Here's how the part is built. I have some questions about the finished solid (model axes, mm). A direction names the side the tool comes from. Round coordinates to 2 decimals unless told otherwise and drop trailing zeros. Loops run counter-clockwise (first coordinate to the right, second up) from the corner with the lowest first, then second, coordinate; pieces in that order, holes last. Notation, with made-up numbers: M 33.5,7.5 L 88.5,7.5 A26 cw 88.5,27.5 Z; hole C -3,-8 d11. An arc over 180 degrees is marked long. Write each question's results on one line, items separated by ' | '. Start each with the question number.
```python
from build123d import *

# Parameters (mm, degrees)
EXTRUDE_1_DEPTH     = 40
CUT_EXTRUDE_1_DEPTH = 47.165463282
SKETCH_4_R          = 2
CUT_EXTRUDE_2_DEPTH = 47.165463282
SKETCH_5_W          = 15
SKETCH_5_H          = 15
EXTRUDE_2_DEPTH     = 17.5


with BuildPart() as part:
    # 草图1 → 凸台-拉伸1 (new body)
    with BuildSketch(Plane.XY):
        Polygon((0, 0), (15, 0), (15, -4), (-4, -4), (-4, 17.5), (0, 17.5), align=None)
    extrude(amount=EXTRUDE_1_DEPTH)

    # 草图2 → 切除-拉伸1 (cut, through all)
    with BuildSketch(Plane(origin=(0, 0, 0), x_dir=(1, 0, 0), z_dir=(0, 1, 0))):
        with BuildLine():
            Line((9.5, -36.5), (5.5, -36.5))
            ThreePointArc((5.5, -36.5), (4, -35), (5.5, -33.5))
            Line((5.5, -33.5), (9.5, -33.5))
            ThreePointArc((9.5, -33.5), (11, -35), (9.5, -36.5))
        make_face()
        with BuildLine():
            Line((9.5, -3.5), (5.5, -3.5))
            ThreePointArc((5.5, -3.5), (4, -5), (5.5, -6.5))
            Line((5.5, -6.5), (9.5, -6.5))
            ThreePointArc((9.5, -6.5), (11, -5), (9.5, -3.5))
        make_face()
    extrude(amount=-CUT_EXTRUDE_1_DEPTH, mode=Mode.SUBTRACT)

    # 草图4 → 切除-拉伸2 (cut, through all)
    with BuildSketch(Plane(origin=(0, 0, 0), x_dir=(0, 0, -1), z_dir=(1, 0, 0))):
        with Locations((-35, 8.75)):
            Circle(SKETCH_4_R)
        with Locations(Location((-5, 8.75, 0), (0, 0, 180))):
            Circle(SKETCH_4_R)
    extrude(amount=-CUT_EXTRUDE_2_DEPTH, mode=Mode.SUBTRACT)

    # 草图5 → 凸台-拉伸2 (add)
    with BuildSketch(Plane(origin=(0, 0, 0), x_dir=(1, 0, 0), z_dir=(0, 1, 0))):
        with Locations((7.5, -20)):
            Rectangle(SKETCH_5_W, SKETCH_5_H)
    extrude(amount=EXTRUDE_2_DEPTH)


solid = part.part
```
1. I want a section at D-D on x = 7.5. List the corners of the cut face in (y, z) for me.
2. I want a section at A-A on z = 5. List the corners of the cut face in (x, y) for me, plus the area to 3 significant figures.
3. I need wall thicknesses on line 1 along Y through (x, z) = (-1.2, 35); line 2 along X through (y, z) = (3.5, 2); line 3 along Z through (x, y) = (13.5, 4.5). Which ranges of each line are inside material? Lowest first, please.
4. If we mould it in two halves opening along X, with no side actions, what happens to faces 5 (the face through (-4, 7, 20)), 6 (the face through (11, -2, 35)), 7 (the face through (7, 0, 32))? For each: released by +X, released by -X, zero draft, split by the parting line, or undercut.
5. For pin 1 (3 mm diameter, centred on x = 8.5, y = -2.5, fed in from -Z); pin 2 (4 mm diameter, centred on x = 10, z = 5, fed in from +Y); pin 3 (10 mm diameter, centred on y = 10, z = 6, fed in from +X); pin 4 (4.5 mm diameter, centred on x = 9, y = 10, fed in from +Z), each with a flat end and sliding along its axis, tell me the tip position at first contact or that it passes through.
6. I want a section at B-B on y = 8.75. List the corners of the cut face in (x, z) for me.
7. Which directions (+Z, -Z, +X, -X, +Y, -Y) give clear straight access to the entire face, cutting with the end or side of a thin tool? Please do faces 1 (the face through (-1, 2, 40)), 2 (the face through (4, -2, 35)), 3 (the face through (0, 9, 8)), 4 (the face through (0, 9, 32)).
8. I want a section at C-C on x = 1.25. List the corners of the cut face in (y, z) for me.
Outcome:
1) outline: M -4,0 L 0,0 L 0,3.5 L -4,3.5 Z; M -4,6.5 L 0,6.5 L 0,12.5 L 17.5,12.5 L 17.5,27.5 L 0,27.5 L 0,33.5 L -4,33.5 Z; M -4,36.5 L 0,36.5 L 0,40 L -4,40 Z
2) outline: M -4,-4 L 4,-4 L 4,0 L 0,0 L 0,6.75 L -4,6.75 Z; M -4,10.75 L 0,10.75 L 0,17.5 L -4,17.5 Z; M 11,-4 L 15,-4 L 15,0 L 11,0 Z | area: 102 mm2
3) line 1: -4 to 6.75, 10.75 to 17.5 | line 2: -4 to 0 | line 3: 12.5 to 27.5
4) face 5: released by -X | face 6: undercut | face 7: zero draft
5) pin 1: z = 0 | pin 2: y = 0 | pin 3: x = 0 | pin 4: z = 27.5
6) outline: M -4,0 L 0,0 L 0,3 L -4,3 Z; M -4,7 L 0,7 L 0,12.5 L 15,12.5 L 15,27.5 L 0,27.5 L 0,33 L -4,33 Z; M -4,37 L 0,37 L 0,40 L -4,40 Z
7) face 1: +Z, +X, -X, +Y, -Y | face 2: +Y, -Y | face 3: -Z, +X, +Y | face 4: +Z, +X, +Y
8) outline: M -4,0 L 0,0 L 0,12.5 L 17.5,12.5 L 17.5,27.5 L 0,27.5 L 0,40 L -4,40 Z
